Autodesk Inventor part; units mm, degrees
ref_plane "YZ Plane" through (0, 0, 0) normal (1, 0, 0) x (0, 1, 0)
ref_plane "XZ Plane" through (0, 0, 0) normal (0, 1, 0) x (-1, 0, 0)
ref_plane "XY Plane" through (0, 0, 0) normal (0, 0, 1) x (1, 0, 0)
sketch "Sketch1" plane through (0, 0, 0) normal (0, 0, 1) x (1, 0, 0)
  circle A0 centre (0, 0) radius 45
  circle A1 centre (0, 0) radius 65
  circle A2 centre (0, 0) radius 55 construction
  circle A3 centre (0, -55) radius 6
  circle A4 centre (0, 55) radius 2.5
  line L0 (0, 0) -> (0, 34.6858) construction
  circle A5 centre (-43.0007, 34.2919) radius 2.5
  circle A6 centre (43.0007, -34.2919) radius 6
  circle A7 centre (-53.621, -12.2387) radius 2.5
  circle A8 centre (53.621, 12.2387) radius 6
  circle A9 centre (-23.8636, -49.5533) radius 2.5
  circle A10 centre (23.8636, 49.5533) radius 6
  circle A11 centre (23.8636, -49.5533) radius 2.5
  circle A12 centre (-23.8636, 49.5533) radius 6
  circle A13 centre (53.621, -12.2387) radius 2.5
  circle A14 centre (-53.621, 12.2387) radius 6
  circle A15 centre (43.0007, 34.2919) radius 2.5
  circle A16 centre (-43.0007, -34.2919) radius 6
  point P0 (0, 17.3429)
  dimension "d0" = 90
  dimension "d1" = 130
  dimension "d2" = 110
  dimension "d3" = 12
  dimension "d4" = 5
  dimension "d7" = 360
extrude "Extrusion1" add sketch "Sketch1" along normal blind 6
fillet "Fillet1" radius 1 2 edges at (-65, 0, 6) (-65, 0, 0)
properties part number "Component 10(Assembly Ring)"
Source: CAD feature listing. Evaluate the final solid. Frame: model axes, mm. Round coordinates to 2 decimals unless told otherwise and drop trailing zeros. Loops run counter-clockwise (first coordinate to the right, second up) from the corner with the lowest first, then second, coordinate; pieces in that order, holes last.
1. Ray query, L1, parallel to X at y = 12, z = 3.2; L2, parallel to Y at x = 5.5, z = 4.15; L3, parallel to Y at x = 39, z = 4.7. Return the intervals inside material, ascending.
2. Section query B-B on x = 0. Output: boundary loops of the cut face in (y, z), and give its area (3 significant figures).
3. Mould query, pull axis Y, two halves, no side actions, for faces 1 (the cylindrical face through (-43.543, 36.732, 2.958)), 2 (the cylindrical face through (62, -19.52, 2.97)), 3 (the cylindrical face through (-48.995, -34.556, 2.958)), 4 (the flat face through (-19, -42, 6)). Classes: released by +Y, released by -Y, zero draft, split by the parting line, or undercut.
4. Section query A-A on y = 0. Output: boundary loops of the cut face in (x, z), and give its area (3 significant figures).
5. Contact query for flat-ended pins moving along their axis: pin 1 (1.5 mm diameter, centred on y = -31.5, z = 5, fed in from -X); pin 2 (2 mm diameter, centred on x = 13, z = 4, fed in from -Y); pin 3 (3 mm diameter, centred on x = 22.5, z = 4.5, fed in from +Y). Output: stop coordinate, or through.
Answers below:
1. L1: x = -63.88 to -59.62, -47.63 to -43.37, 43.37 to 47.63, 59.62 to 63.88
1. L2: y = -64.77 to -57.4, -52.6 to -44.66, 44.66 to 64.77
1. L3: y = -52 to -38.76, -29.82 to -22.45, 22.45 to 52
2. outline: (-65, 1) arc R1 ccw to (-64, 0) - (-61, 0) - (-61, 6) - (-64, 6) arc R1 ccw to (-65, 5) - close; (-49, 0) - (-45, 0) - (-45, 6) - (-49, 6) - close; (45, 0) - (52.5, 0) - (52.5, 6) - (45, 6) - close; (57.5, 0) - (64, 0) arc R1 ccw to (65, 1) - (65, 5) arc R1 ccw to (64, 6) - (57.5, 6) - close
2. area: 137 mm2
3. face 1: undercut
3. face 2: split by the parting line
3. face 3: undercut
3. face 4: zero draft
4. outline: (-65, 1) arc R1 ccw to (-64, 0) - (-45, 0) - (-45, 6) - (-64, 6) arc R1 ccw to (-65, 5) - close; (45, 0) - (64, 0) arc R1 ccw to (65, 1) - (65, 5) arc R1 ccw to (64, 6) - (45, 6) - close
4. area: 239 mm2
5. pin 1: stops at x = -57.27
5. pin 2: stops at y = -63.88
5. pin 3: stops at y = 61.51
